Design review of the part built by this model. Coordinates are the model's own, in mm. Face numbers are marked on the shaded views. A direction names the side the tool comes from. Give positions to 0.01 mm unless a question says otherwise; leave off trailing zeros. Order: outer loops, then holes, each group sorted by start corner. A loop starts at its lowest first (then second) coordinate and runs counter-clockwise, first axis right, second up. Notation, with made-up numbers: (16, -9.75) -> (57, -9.75) arc R22 cw to (57, 0.25) -> close; hole circle Ø5 at (-32, 29). An arc over 180 degrees is marked (long way). Return JSON: item names as keys, results as strings.
```python
from build123d import *

# Parameters (mm, degrees)
SKETCH1_W                      = 20.955
SKETCH1_H                      = 20.701
BOSS_EXTRUDE1_DEPTH            = 7.62
FILLET3_R                      = 0.762
SHELL1_T                       = -1.016
SKETCH3_W                      = 18.923
SKETCH3_H                      = 1.016
CUT_EXTRUDE1_DEPTH             = 6.604
CONVERT_SOLID1_START           = -10.4775
CONVERT_SOLID1_OUTLINE_W       = 20.701
CONVERT_SOLID1_OUTLINE_H       = 6.604
CONVERT_SOLID1_DEPTH           = 20.955
CONVERT_SOLID1_2_OUTLINE_W     = 20.701
CONVERT_SOLID1_2_OUTLINE_H     = 1.016
CONVERT_SOLID1_2_DEPTH         = 0.762
CONVERT_SOLID1_START_2         = 9.7155
CONVERT_SOLID1_3_OUTLINE_W     = 20.701
CONVERT_SOLID1_3_OUTLINE_H     = 1.016
CONVERT_SOLID1_3_DEPTH         = 0.762
EDGE_FLANGE1_STRIP_W           = 6.096
EDGE_FLANGE1_STRIP_H           = 1.016
EDGE_FLANGE1_STRIP_CUT_DEPTH   = 20.701
EDGE_FLANGE1_STRIP_2_W         = 6.096
EDGE_FLANGE1_STRIP_2_H         = 1.016
EDGE_FLANGE1_STRIP_CUT_2_DEPTH = 20.701
EDGE_FLANGE1_DEPTH             = 20.701
EDGE_FLANGE1_BEND_DEPTH        = 20.701
EDGE_FLANGE2_DEPTH             = 17.399
CHAMFER1_SIZE                  = 2.54
SKETCH23_W                     = 15.399
SKETCH23_H                     = 17.526
CUT_EXTRUDE2_DEPTH             = 20.071990326
FILLET5_R                      = 1.27
SKETCH24_W                     = 1
SKETCH24_H                     = 17.526
SKETCH24_W_2                   = 15.399
SKETCH24_H_2                   = 1
EXTRUDE_THIN1_DEPTH            = 1.016
BOSS_EXTRUDE2_DEPTH            = 3.302
FILLET4_R                      = 2.54
F_3_5_3_5_DIAMETER_HOLE1_D     = 3.5
FILLET6_R                      = 2.54


with BuildPart() as part:
    # Sketch1 → Boss-Extrude1 (new body)
    with BuildSketch(Plane.XY):
        Rectangle(SKETCH1_W, SKETCH1_H)
    extrude(amount=BOSS_EXTRUDE1_DEPTH)

    # Fillet3
    fillet3_edges = [part.edges().sort_by_distance(p)[0] for p in [
        (10.4775, 0, 7.62),
        (-10.4775, 0, 7.62),
    ]]
    fillet(fillet3_edges, radius=FILLET3_R)

    # Shell1
    shell1_openings = [part.faces().sort_by_distance(p)[0] for p in [
        (0, 0, 0),
    ]]
    offset(amount=SHELL1_T, openings=shell1_openings, kind=Kind.INTERSECTION)

    # Sketch3 → Cut-Extrude1 (cut)
    with BuildSketch(Plane(origin=(0, 0, 0), x_dir=(-1, 0, 0), z_dir=(0, 0, -1))):
        with Locations((0, -9.8425)):
            Rectangle(SKETCH3_W, SKETCH3_H)
    extrude(amount=-CUT_EXTRUDE1_DEPTH, mode=Mode.SUBTRACT)

    # Convert-Solid1: read off the stored shape, not the designer's step
    # Convert-Solid1 outline → Convert-Solid1 (cut)
    with BuildSketch(Plane.YZ.offset(CONVERT_SOLID1_START)):
        with Locations((0, 3.302)):
            Rectangle(CONVERT_SOLID1_OUTLINE_W, CONVERT_SOLID1_OUTLINE_H)
    extrude(amount=CONVERT_SOLID1_DEPTH, mode=Mode.SUBTRACT)

    # Convert-Solid1 2 outline → Convert-Solid1 2 (cut)
    with BuildSketch(Plane.YZ.offset(CONVERT_SOLID1_START)):
        with Locations((0, 7.112)):
            Rectangle(CONVERT_SOLID1_2_OUTLINE_W, CONVERT_SOLID1_2_OUTLINE_H)
    extrude(amount=CONVERT_SOLID1_2_DEPTH, mode=Mode.SUBTRACT)

    # Convert-Solid1 3 outline → Convert-Solid1 3 (cut)
    with BuildSketch(Plane.YZ.offset(CONVERT_SOLID1_START_2)):
        with Locations((0, 7.112)):
            Rectangle(CONVERT_SOLID1_3_OUTLINE_W, CONVERT_SOLID1_3_OUTLINE_H)
    extrude(amount=CONVERT_SOLID1_3_DEPTH, mode=Mode.SUBTRACT)

    # Edge-Flange1: sheet metal written as solids
    # Edge-Flange1 strip (on a plane across the edge) → Edge-Flange1 strip cut (cut)
    with BuildSketch(Plane(origin=(9.7155, 10.3505, 6.604), x_dir=(-1, 0, 0), z_dir=(0, -1, 0))):
        with Locations((-2.032, -0.508)):
            Rectangle(EDGE_FLANGE1_STRIP_W, EDGE_FLANGE1_STRIP_H)
    extrude(amount=EDGE_FLANGE1_STRIP_CUT_DEPTH, mode=Mode.SUBTRACT)

    # Edge-Flange1 strip 2 (on a plane across the edge) → Edge-Flange1 strip cut 2 (cut)
    with BuildSketch(Plane(origin=(-9.7155, -10.3505, 6.604), x_dir=(1, 0, 0), z_dir=(0, 1, 0))):
        with Locations((-2.032, -0.508)):
            Rectangle(EDGE_FLANGE1_STRIP_2_W, EDGE_FLANGE1_STRIP_2_H)
    extrude(amount=EDGE_FLANGE1_STRIP_CUT_2_DEPTH, mode=Mode.SUBTRACT)

    # Edge-Flange1 section (on a plane across the edge) → Edge-Flange1 (add)
    with BuildSketch(Plane(origin=(9.7155, 10.3505, 6.604), x_dir=(-1, 0, 0), z_dir=(0, -1, 0))):
        with BuildLine():
            Line((-1.016, 1.016), (-1.016, 6.8834))
            Line((-1.016, 6.8834), (0, 6.8834))
            Line((0, 6.8834), (0, 1.016))
            ThreePointArc((0, 1.016), (0.29757951, 0.29757951), (1.016, 0))
            Line((1.016, 0), (1.016, -1.016))
            ThreePointArc((1.016, -1.016), (-0.420840979, -0.420840979), (-1.016, 1.016))
        make_face()
    extrude(amount=EDGE_FLANGE1_DEPTH)

    # Edge-Flange1 section 2 (on a plane across the edge) → Edge-Flange1 bend (add)
    with BuildSketch(Plane(origin=(-9.7155, -10.3505, 6.604), x_dir=(1, 0, 0), z_dir=(0, 1, 0))):
        with BuildLine():
            Line((-1.016, 1.016), (-1.016, 6.8834))
            Line((-1.016, 6.8834), (0, 6.8834))
            Line((0, 6.8834), (0, 1.016))
            ThreePointArc((0, 1.016), (0.29757951, 0.29757951), (1.016, 0))
            Line((1.016, 0), (1.016, -1.016))
            ThreePointArc((1.016, -1.016), (-0.420840979, -0.420840979), (-1.016, 1.016))
        make_face()
    extrude(amount=EDGE_FLANGE1_BEND_DEPTH)

    # Edge-Flange2: sheet metal written as solids
    # Edge-Flange2 section (on a plane across the edge) → Edge-Flange2 (add)
    with BuildSketch(Plane(origin=(8.6995, -10.62273638, 6.604), x_dir=(0, 0.49999999999999495, -0.8660254037844416), z_dir=(-1, 0, 0))):
        with BuildLine():
            Line((-1.016, 0.27223638), (-1.016, 2.90276362))
            Line((-1.016, 2.90276362), (0, 2.90276362))
            Line((0, 2.90276362), (0, 0.27223638))
            ThreePointArc((0, 0.27223638), (0.03461936, 0.00927623), (0.13611819, -0.23576362))
            Line((0.13611819, -0.23576362), (-0.74376362, -0.74376362))
            ThreePointArc((-0.74376362, -0.74376362), (-0.946761279, -0.25368392), (-1.016, 0.27223638))
        make_face()
    extrude(amount=EDGE_FLANGE2_DEPTH)

    # Chamfer1
    chamfer1_edges = [part.edges().sort_by_distance(p)[0] for p in [
        (8.6995, -13.390603416, 5.592559095),
        (-8.6995, -13.390603416, 5.592559095),
    ]]
    chamfer(chamfer1_edges, length=CHAMFER1_SIZE)

    # Sketch23 → Cut-Extrude2 (cut, through all)
    with BuildSketch(Plane.XY.offset(7.62)):
        Rectangle(SKETCH23_W, SKETCH23_H)
    extrude(amount=-CUT_EXTRUDE2_DEPTH, mode=Mode.SUBTRACT)

    # Fillet5
    fillet5_edges = [part.edges().sort_by_distance(p)[0] for p in [
        (-7.6995, 8.763, 7.112),
        (7.6995, 8.763, 7.112),
        (7.6995, -8.763, 7.112),
        (-7.6995, -8.763, 7.112),
    ]]
    fillet(fillet5_edges, radius=FILLET5_R)

    # Sketch24 → Extrude-Thin1 (add)
    with BuildSketch(Plane.XY.offset(7.62)):
        Rectangle(SKETCH24_W, SKETCH24_H)
        with Locations((0, -4.953)):
            Rectangle(SKETCH24_W_2, SKETCH24_H_2)
        with Locations((0, 4.953)):
            Rectangle(SKETCH24_W_2, SKETCH24_H_2)
    extrude(amount=-EXTRUDE_THIN1_DEPTH)

    # Sketch25 → Boss-Extrude2 (add)
    with BuildSketch(Plane(origin=(0, 10.3505, 0), x_dir=(1, 0, 0), z_dir=(0, 1, 0))):
        with BuildLine():
            Line((10.7315, -5.588), (10.7315, 0.2794))
            Line((10.7315, 0.2794), (9.7155, 0.2794))
            Line((9.7155, 0.2794), (9.7155, -5.588))
            ThreePointArc((9.7155, -5.588), (9.41792049, -6.30642049), (8.6995, -6.604))
            Line((8.6995, -6.604), (-8.6995, -6.604))
            ThreePointArc((-8.6995, -6.604), (-9.41792049, -6.30642049), (-9.7155, -5.588))
            Line((-9.7155, -5.588), (-9.7155, 0.2794))
            Line((-9.7155, 0.2794), (-10.7315, 0.2794))
            Line((-10.7315, 0.2794), (-10.7315, -5.588))
            ThreePointArc((-10.7315, -5.588), (-10.136340979, -7.024840979), (-8.6995, -7.62))
            Line((-8.6995, -7.62), (8.6995, -7.62))
            ThreePointArc((8.6995, -7.62), (10.136340979, -7.024840979), (10.7315, -5.588))
        make_face()
    extrude(amount=BOSS_EXTRUDE2_DEPTH)

    # Fillet4
    fillet4_edges = [part.edges().sort_by_distance(p)[0] for p in [
        (10.2235, 13.6525, -0.2794),
        (-10.2235, 13.6525, -0.2794),
        (10.2235, -10.3505, -0.2794),
        (-10.2235, -10.3505, -0.2794),
    ]]
    fillet(fillet4_edges, radius=FILLET4_R)

    # Ø3.5 (3.5) Diameter Hole1 (through all)
    with Locations(Plane(origin=(10.7315, 0, 0), x_dir=(0, 0, -1), z_dir=(1, 0, 0))):
        with Locations((-3.5386, 11.8745)):
            Hole(F_3_5_3_5_DIAMETER_HOLE1_D / 2)

    # Fillet6
    fillet6_edges = [part.edges().sort_by_distance(p)[0] for p in [
        (-6.1595, -13.390603416, 5.592559095),
        (6.1595, -13.390603416, 5.592559095),
    ]]
    fillet(fillet6_edges, radius=FILLET6_R)


solid = part.part
```
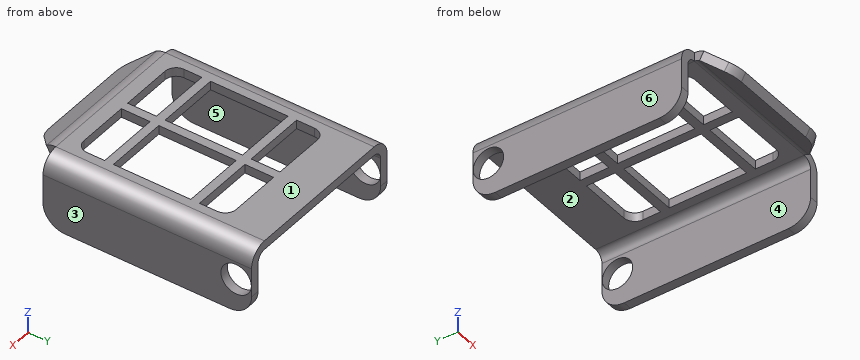
Item 1: Machinability: for the marked faces 5 and 6, which of the approach directions +Z, -Z, +X, -X, +Y, -Y give a long, thin tool a straight path to every point of the face, cutting with its end or side? Answer none if there is none.
Result set:
{"face 5": "-Z, +Y, -Y", "face 6": "+Z, -Z, -X, +Y, -Y"}
Item 2: For pin 1 (0.8 mm diameter, centred on y = 7.5, z = 7, fed in from +X); pin 2 (1.1 mm diameter, centred on y = 2, z = 7, fed in from -X); pin 3 (1.2 mm diameter, centred on y = -11, z = 7, fed in from +X), all flat-tipped, find the tip position at first contact; note any pin that passes through.
Result set:
{"pin 1": "stops at x = 10.46", "pin 2": "stops at x = -10.54", "pin 3": "stops at x = 8.7"}
Item 3: Mouldability with a two-part tool opening along X and no side actions: class the marked faces 1, 2, 3 and 4 as released by +X, released by -X, zero draft, split by the parting line, or undercut.
Result set:
{"face 1": "zero draft", "face 2": "undercut", "face 3": "released by +X", "face 4": "undercut"}
Item 4: Add section C-C (z = 3). Give the boundary of the cut face in (x, y), plus the area to 3 significant figures.
Result set:
{"outline": "(-10.73, -10.35) -> (-9.72, -10.35) -> (-9.72, 10.21) -> (-10.73, 10.21) -> close; (-10.73, 13.54) -> (-9.72, 13.54) -> (-9.72, 13.65) -> (-10.73, 13.65) -> close; (9.72, -10.35) -> (10.73, -10.35) -> (10.73, 10.21) -> (9.72, 10.21) -> close; (9.72, 13.54) -> (10.73, 13.54) -> (10.73, 13.65) -> (9.72, 13.65) -> close", "area": "42.0 mm^2"}
Item 5: Add section A-A (y = -3.75). Give the boundary of the cut face in (x, z).
Result set:
{"outline": "(-10.73, -0.28) -> (-9.72, -0.28) -> (-9.72, 5.59) arc R1.02 cw to (-8.7, 6.6) -> (-7.7, 6.6) -> (-7.7, 7.62) -> (-8.7, 7.62) arc R2.03 ccw to (-10.73, 5.59) -> close; (-0.5, 6.6) -> (0.5, 6.6) -> (0.5, 7.62) -> (-0.5, 7.62) -> close; (7.7, 6.6) -> (8.7, 6.6) arc R1.02 cw to (9.72, 5.59) -> (9.72, -0.28) -> (10.73, -0.28) -> (10.73, 5.59) arc R2.03 ccw to (8.7, 7.62) -> (7.7, 7.62) -> close"}
Item 6: Add section B-B (x = 3.5). Give the boundary of the cut face in (y, z), plus the area to 3 significant figures.
Result set:
{"outline": "(-13.64, 6.03) -> (-13.14, 5.15) -> (-10.86, 6.47) arc R1.02 cw to (-10.35, 6.6) -> (-8.76, 6.6) -> (-8.76, 7.62) -> (-10.35, 7.62) arc R2.03 ccw to (-11.37, 7.35) -> close; (-5.45, 6.6) -> (-4.45, 6.6) -> (-4.45, 7.62) -> (-5.45, 7.62) -> close; (4.45, 6.6) -> (5.45, 6.6) -> (5.45, 7.62) -> (4.45, 7.62) -> close; (8.76, 6.6) -> (13.65, 6.6) -> (13.65, 7.62) -> (8.76, 7.62) -> close", "area": "12.1 mm^2"}
Item 7: Add section D-D (y = 9.75). Give the boundary of the cut face in (x, z), plus the area to 3 significant figures.
Result set:
{"outline": "(-10.73, -0.28) -> (-9.72, -0.28) -> (-9.72, 5.59) arc R1.02 cw to (-8.7, 6.6) -> (8.7, 6.6) arc R1.02 cw to (9.72, 5.59) -> (9.72, -0.28) -> (10.73, -0.28) -> (10.73, 5.59) arc R2.03 ccw to (8.7, 7.62) -> (-8.7, 7.62) arc R2.03 ccw to (-10.73, 5.59) -> close", "area": "34.5 mm^2"}
Item 8: Wall thickness on L1, parallel to X at y = -9.75, z = 4; L2, parallel to X at y = 6.5, z = 6; L3, parallel to Z at x = -0.25, y = -3.25: over which ranges is each line inside the solid? List them lowest first. Write a range as [from, to].
Result set:
{"L1": "x = [-10.73, -9.72], [9.72, 10.73]", "L2": "x = [-10.69, -9.63], [9.63, 10.69]", "L3": "z = [6.6, 7.62]"}
